CAD build for the part. Positions are in the model's coordinates, mm. A direction names the side the tool comes from. Coordinates: 2 decimals unless noted, no trailing zeros. Write each loop counter-clockwise with the first axis right and the second up, starting at its lowest first coordinate (ties: lowest second). Pieces come first, ordered by that corner, then holes. Notation, with made-up numbers: (-40, 65) - (-4, 65) arc R25 ccw to (-4, 77) - close; hole circle Ø3 at (78, 1.25). An arc over 180 degrees is marked (long way). Answer in a Markdown table with one row per item. Add a question column.
Q1. 3-axis set-ups, long thin cutter, end or side, ignore diameter. For faces 1 (the flat face through (26.62, -22.09, 31.27)), 2 (the cylindrical face through (-52.6, -29.6, 54.5)), 3 (the flat face through (-21, -35, -37.5)), 4 (the flat face through (25, -9, 21)): which of +Z, -Z, +X, -X, +Y, -Y reach the whole face in a straight line?
Q2. Band-saw the part on D-D (x = 13.5). State how many separate pieces and enclosed holes the cut face has, and give its area (3 significant figures).
Q3. Band-saw the part on B-B (x = -41). List the corners of the cut face in (y, z).
Q4. Band-saw the part on C-C (z = 26.75). List the corners of the cut face in (x, y).
Q5. Pin check, flat tips, straight feed: pin 1 (0.9 mm diameter, centred on x = 55.5, z = 11.5, fed in from -Y); pin 2 (3.5 mm diameter, centred on x = 8, z = -12.5, fed in from -Y); pin 3 (1.5 mm diameter, centred on x = 7, z = 1, fed in from -Y). Stop position of each tip, or through.
Q6. Two-plate mould, pull along Y, no slides. Class faces 5 (the flat face through (-23, -60, 0)), 6 (the flat face through (-60, -30, -57)), 7 (the flat face through (25, -5, 0)): +Y half, -Y half, draft (parallel to the pull), parting line (faces both ways), or undercut.
Q7. Drill centre lines: line 1 along Y through (x, z) = (13, -18); line 2 along Y through (x, z) = (13.5, 30.9); line 3 along Z through (x, y) = (42, -8.5). Where is each one in solid material? Low to high. Write a range as from..to.
Q8. Band-saw the part on A-A (y = -45). List the corners of the cut face in (x, z).
Autodesk Inventor part; units mm, degrees
ref_plane "YZ Plane" through (0, 0, 0) normal (1, 0, 0) x (0, 1, 0)
ref_plane "XZ Plane" through (0, 0, 0) normal (0, 1, 0) x (-1, 0, 0)
ref_plane "XY Plane" through (0, 0, 0) normal (0, 0, 1) x (1, 0, 0)
sketch "Boceto2" plane through (0, 0, 0) normal (0, 1, 0) x (-1, 0, 0)
  line L0 (60, -60) -> (15.6267, -60)
  line L1 (15.6267, 60) -> (60, 60)
  arc A0 (45.1786, 52.9653) -> (45.1786, -52.9653) centre (130, 0) ccw
  arc A1 (45.1786, -52.9653) -> (60, -55) centre (60, 0) ccw
  arc A2 (60, 55) -> (45.1786, 52.9653) centre (60, 0) ccw
  line L2 (60, 60) -> (60, 55)
  line L3 (60, -55) -> (60, -60)
  line L4 (5, 32.5) -> (-60, 32.5)
  line L5 (5, -32.5) -> (-60, -32.5)
  line L6 (-60, -32.5) -> (-60, 32.5)
  arc A3 (15.6267, 60) -> (5, 32.5) centre (130, 0) ccw
  arc A4 (5, -32.5) -> (15.6267, -60) centre (130, 0) ccw
  line L7 (-60, 0) -> (60, 0) construction
  point P0 (0, 0)
  point P1 (30, 0)
  dimension "d8" = 200
  dimension "d13" = 65
  dimension "d17" = 65
  dimension "d18" = 65
  dimension "d19" = 30
extrude "Extrusión1" add sketch "Boceto2" against normal blind 60
sketch "Boceto4" plane through (0, -60, 0) normal (0, -1, 0) x (1, 0, 0)
  line L0 (60, -32.5) -> (60, 32.5)
  line L1 (60, -30) -> (60, 30)
  arc A0 (-24.1699, -30) -> (-24.1699, 30) centre (-130, 0) ccw
  arc A1 (-45.1786, -52.9653) -> (-45.1786, 52.9653) centre (-130, 0) ccw
  line L2 (-24.1699, -30) -> (60, -30)
  line L3 (60, 30) -> (-24.1699, 30)
  point P0 (0, 0)
  point P1 (-40, 0)
  point P2 (-30, 0)
  dimension "d26" = 100
  dimension "d27" = 220
  dimension "d28" = 60
extrude "Extrusión2" cut sketch "Boceto4" against normal blind 45
sketch "Boceto5" plane through (-5, 0, 32.5) normal (0, 0, 1) x (1, 0, 0)
  line L0 (65, 0) -> (65, -60)
  line L1 (65, -60) -> (0, -60)
  line L2 (38.5, -26.2) -> (0, -26.2) construction
  line L3 (0, 0) -> (0, -60)
  arc A0 (26.666, -23.8432) -> (26.7187, -28.5748) centre (27.5, -26.2) ccw
  line L4 (36.4416, -20.3837) -> (26.666, -23.8432)
  line L5 (36.6445, -31.8401) -> (26.7187, -28.5748)
  line L6 (65, -29.7625) -> (43.25, -29.7625)
  line L7 (43.25, -22.2625) -> (65, -22.2625)
  line L8 (65, -22.2625) -> (65, -29.7625)
  arc A1 (36.6445, -31.8401) -> (43.25, -29.7625) centre (38.5, -26.2) ccw
  arc A2 (43.25, -22.2625) -> (36.4416, -20.3837) centre (38.5, -26.2) ccw
  circle A3 centre (18.5, -35.45) radius 1.4875
  circle A4 centre (18.5, -16.95) radius 1.4875
  point P0 (5, 0)
  point P1 (44.75, -26.2)
  dimension "d29" = 26.5
  dimension "d31" = 33.8
  dimension "d32" = 5
  dimension "d33" = 11
  dimension "d34" = 7.5
  dimension "d38" = 46.5
  dimension "d39" = 24.55
  dimension "d40" = 2.975
extrude "Extrusión3" cut sketch "Boceto5" against normal blind 65
sketch "Boceto7" plane through (0, -60, 0) normal (0, -1, 0) x (1, 0, 0)
  arc A0 (-24.1699, -30) -> (-24.1699, 30) centre (-130, 0) ccw
  line L0 (60, -30) -> (-24.1699, -30)
  line L1 (-24.1699, 30) -> (60, 30)
  line L2 (60, 30) -> (60, -30)
  point P0 (0, 0)
extrude "Extrusión4" add sketch "Boceto7" against normal blind 22
sketch "Boceto8" plane through (0, -60, 0) normal (0, -1, 0) x (1, 0, 0)
  line L0 (60, -30) -> (-24.1699, -30)
  arc A0 (-24.1699, -30) -> (-24.1699, 30) centre (-130, 0) ccw
  line L1 (-24.1699, 30) -> (60, 30)
  line L2 (60, -30) -> (60, 30)
  point P0 (0, 0)
extrude "Extrusión5" cut sketch "Boceto8" against normal blind 19.5
sketch "Boceto9" plane through (0, -40.5, 0) normal (0, -1, 0) x (1, 0, 0)
  line L0 (60, 8.5) -> (60, -8.5)
  arc A0 (-20.3289, -8.5) -> (-20.3289, 8.5) centre (-130, 0) ccw
  line L1 (60, 30) -> (60, -30)
  line L2 (60, -8.5) -> (-20.3289, -8.5)
  line L3 (60, 8.5) -> (-20.3289, 8.5)
  point P0 (0, 0)
  point P1 (60, -10)
  point P2 (60, 10)
  point P3 (-30, 0)
  dimension "d52" = 8.5
  dimension "d53" = 8.5
extrude "Extrusión6" cut sketch "Boceto9" against normal blind 2.5
sketch "Boceto10" plane through (0, -40.5, 0) normal (0, -1, 0) x (1, 0, 0)
  line L0 (55, 11.75) -> (8.5, 11.75) construction
  line L1 (8.5, 11.75) -> (8.5, -11.75) construction
  line L2 (8.5, -11.75) -> (55, -11.75) construction
  line L3 (55, -11.75) -> (55, 11.75) construction
  line L4 (60, 30) -> (60, 8.5) construction
  line L5 (-20.3289, 8.5) -> (60, 8.5) construction
  line L6 (58.25, 15) -> (51.75, 15)
  line L7 (51.75, 15) -> (51.75, 8.5)
  line L8 (51.75, 8.5) -> (58.25, 8.5)
  line L9 (58.25, 8.5) -> (58.25, 15)
  line L10 (58.25, 15) -> (51.75, 8.5) construction
  line L11 (51.75, 15) -> (58.25, 8.5) construction
  line L12 (60, -8.5) -> (-20.3289, -8.5) construction
  line L13 (58.25, -15) -> (51.75, -15)
  line L14 (51.75, -15) -> (51.75, -8.5)
  line L15 (51.75, -8.5) -> (58.25, -8.5)
  line L16 (58.25, -8.5) -> (58.25, -15)
  line L17 (58.25, -15) -> (51.75, -8.5) construction
  line L18 (51.75, -15) -> (58.25, -8.5) construction
  line L19 (5.25, -15) -> (11.75, -15)
  line L20 (11.75, -15) -> (11.75, -8.5)
  line L21 (11.75, -8.5) -> (5.25, -8.5)
  line L22 (5.25, -8.5) -> (5.25, -15)
  line L23 (5.25, -15) -> (11.75, -8.5) construction
  line L24 (11.75, -15) -> (5.25, -8.5) construction
  line L25 (11.75, 15) -> (5.25, 15)
  line L26 (5.25, 15) -> (5.25, 8.5)
  line L27 (5.25, 8.5) -> (11.75, 8.5)
  line L28 (11.75, 8.5) -> (11.75, 15)
  line L29 (11.75, 15) -> (5.25, 8.5) construction
  line L30 (5.25, 15) -> (11.75, 8.5) construction
  point P0 (0, 0)
  point P1 (8.5, 0)
  dimension "d50" = 46.5
  dimension "d51" = 23.5
  dimension "d54" = 5
  dimension "d55" = 6.5
  dimension "d56" = 6.5
extrude "Extrusión7" add sketch "Boceto10" along normal blind 2.5
sketch "Boceto11" plane through (0, -43, 0) normal (0, -1, 0) x (1, 0, 0)
  line L0 (5.25, 8.5) -> (11.75, 8.5) construction
  line L1 (5.25, 8.5) -> (5.25, 11.75) construction
  line L2 (5.25, 8.5) -> (5.25, 15) construction
  line L3 (11.75, 8.5) -> (11.75, 15) construction
  line L4 (11.75, 11.75) -> (5.25, 11.75) construction
  line L5 (8.5, 11.75) -> (55, 11.75) construction
  line L6 (55, 11.75) -> (55, -11.75) construction
  line L7 (55, -11.75) -> (8.5, -11.75) construction
  line L8 (8.5, -11.75) -> (8.5, 11.75) construction
  circle A0 centre (8.5, 11.75) radius 1.5
  circle A1 centre (8.5, -11.75) radius 1.5
  circle A2 centre (55, 11.75) radius 1.5
  circle A3 centre (55, -11.75) radius 1.5
  point P0 (0, 0)
  dimension "d59" = 46.5
  dimension "d60" = 23.5
  dimension "d62" = 3
extrude "Extrusión8" cut sketch "Boceto11" against normal blind 4
sketch "Boceto12" plane through (0, -60, 0) normal (0, -1, 0) x (1, 0, 0)
  arc A0 (-45.1786, -52.9653) -> (-45.1786, 52.9653) centre (-130, 0) ccw
  line L0 (-60, -60) -> (-15.6267, -60)
  line L1 (-23.3464, -55) -> (-34.7372, -55)
  arc A1 (-5, 32.5) -> (-15.6267, 60) centre (-130, 0) ccw
  line L2 (-23.3464, 55) -> (-34.7372, 55)
  arc A2 (-15.6267, -60) -> (-5, -32.5) centre (-130, 0) ccw
  arc A3 (-26.5894, 37.5) -> (-34.7372, 55) centre (-130, 0) ccw
  arc A4 (-34.7372, -55) -> (-26.5894, -37.5) centre (-130, 0) ccw
  arc A5 (-16.0099, 37.5) -> (-23.3464, 55) centre (-130, 0) ccw
  arc A6 (-23.3464, -55) -> (-16.0099, -37.5) centre (-130, 0) ccw
  line L3 (-16.0099, 37.5) -> (-26.5894, 37.5)
  line L4 (-16.0099, -37.5) -> (-26.5894, -37.5)
  point P0 (0, 0)
extrude "Extrusión9" cut sketch "Boceto12" against normal blind 50
sketch "Boceto14" plane through (60, 0, 32.5) normal (1, 0, 0) x (0, 0, -1)
  line L0 (65, 0) -> (65, -22.2625) construction
  line L1 (0, 0) -> (0, -60) construction
  line L2 (65, -5) -> (0, -5) construction
  line L3 (0, -6.25) -> (0, -11.25)
  line L4 (0, -12.5) -> (65, -12.5) construction
  line L5 (65, -11.25) -> (65, -6.25)
  line L6 (0, 0) -> (65, 0) construction
  line L7 (2.5, -15) -> (62.5, -15) construction
  line L8 (53.5, -5) -> (11.5, -5)
  line L9 (11.5, -12.5) -> (53.5, -12.5)
  line L10 (0, -6.25) -> (0, -11.25)
  line L11 (65, -11.25) -> (65, -6.25)
  line L12 (65, -6.25) -> (53.5, -6.25)
  line L13 (11.5, -6.25) -> (0, -6.25)
  line L14 (0, -11.25) -> (11.5, -11.25)
  line L15 (53.5, -11.25) -> (65, -11.25)
  line L16 (53.5, -12.5) -> (53.5, -11.25)
  line L17 (53.5, -6.25) -> (53.5, -5)
  line L18 (11.5, -5) -> (11.5, -6.25)
  line L19 (11.5, -11.25) -> (11.5, -12.5)
  point P0 (32.5, 0)
  point P1 (32.5, -5)
  point P2 (32.5, 0)
  dimension "d74" = 5
  dimension "d75" = 2.5
  dimension "d76" = 42
  dimension "d77" = 5
  dimension "d85" = 1.25
  dimension "d86" = 1.25
  dimension "d87" = 5
extrude "Extrusión10" cut sketch "Boceto14" against normal blind 5
sketch "Boceto15" plane through (55, 0, 32.5) normal (1, 0, 0) x (0, 0, -1)
  line L0 (53.5, -12.5) -> (11.5, -12.5)
  line L1 (11.5, -6.25) -> (11.5, -5)
  line L2 (53.5, -12.5) -> (11.5, -12.5)
  line L3 (11.5, -12.5) -> (11.5, -5)
  line L4 (11.5, -5) -> (53.5, -5)
  line L5 (53.5, -5) -> (53.5, -12.5)
  point P0 (32.5, 0)
extrude "Extrusión11" cut sketch "Boceto15" against normal blind 65
sketch "Boceto16" plane through (55, 0, 32.5) normal (1, 0, 0) x (0, 0, -1)
  line L0 (53.5, -6.25) -> (65, -6.25) construction
  line L1 (59.25, -6.25) -> (59.25, -11.25) construction
  line L2 (65, -11.25) -> (53.5, -11.25) construction
  circle A0 centre (59.25, -8.75) radius 1.4875
  line L3 (32.5, 0) -> (32.5, -15) construction
  line L4 (2.5, -15) -> (62.5, -15) construction
  circle A1 centre (5.75, -8.75) radius 1.4875
  dimension "d82" = 2.975
extrude "Extrusión12" cut sketch "Boceto16" against normal blind 7
sketch "Boceto17" plane through (0, 0, 0) normal (0, 1, 0) x (1, 0, 0)
  arc A0 (-45.1786, -52.9653) -> (-45.1786, 52.9653) centre (-130, 0) ccw construction
  line L0 (-5, 32.5) -> (60, 32.5)
  arc A1 (-5, -32.5) -> (-5, 32.5) centre (-130, 0) ccw
  line L1 (60, -32.5) -> (60, 32.5)
  line L2 (-5, -32.5) -> (60, -32.5)
  point P0 (0, 0)
extrude "Extrusión13" cut sketch "Boceto17" against normal blind 2.5
properties part number "Chasis"
Checked values:
| question | item | result |
|---|---|---|
| 1 | face 1 | +Z, -Z |
| 1 | face 2 | -X, +Y, -Y |
| 1 | face 3 | -Y |
| 1 | face 4 | +X |
| 2 | separate pieces | 5 |
| 2 | enclosed holes | 1 |
| 2 | area | 800 mm² |
| 3 | outline | (-60, -60) - (0, -60) - (0, -45.6) - (-60, -45.6) - close; (-60, 45.6) - (0, 45.6) - (0, 60) - (-60, 60) - close |
| 4 | outline | (-33.64, -60) - (-23.3, -60) - (-23.3, -40.5) - (60, -40.5) - (60, -38) - (-23.3, -38) - (-23.3, -15) - (60, -15) - (60, -11.25) - (55, -11.25) - (55, -10.24) - (48, -10.24) - (48, -7.26) - (55, -7.26) - (55, -6.25) - (60, -6.25) - (60, -2.5) - (-3.64, -2.5) - (-3.64, 0) - (-33.64, 0) - close |
| 5 | pin 1 | stops at y = -39 |
| 5 | pin 2 | stops at y = -43 |
| 5 | pin 3 | stops at y = -15 |
| 6 | face 5 | -Y half |
| 6 | face 6 | draft |
| 6 | face 7 | undercut |
| 7 | line 1 | y = -40.5..-38, -15..-12.5, -5..-2.5 |
| 7 | line 2 | y = -60..-36.94, -33.96..-18.44, -15.46..-2.5 |
| 7 | line 3 | z = -32.5..-21, 21..32.5 |
| 8 | outline | (-60, -60) - (-15.63, -60) arc R129.16 ccw to (-5, -32.5) - (60, -32.5) - (60, -30) - (-24.17, -30) arc R110 ccw to (-24.17, 30) - (60, 30) - (60, 32.5) - (-5, 32.5) arc R129.16 ccw to (-15.63, 60) - (-60, 60) - (-60, 55) arc R55 cw to (-45.18, 52.97) arc R100 cw to (-45.18, -52.97) arc R55 cw to (-60, -55) - close; hole (-34.74, -55) - (-23.35, -55) arc R120 ccw to (-16.01, -37.5) - (-26.59, -37.5) arc R110 cw to start; hole (-34.74, 55) arc R110 cw to (-26.59, 37.5) - (-16.01, 37.5) arc R120 ccw to (-23.35, 55) - close |
